```python
from build123d import *

# Parameters (mm, degrees)
CROQUIS1_R                = 3
SALIENTE_EXTRUIR1_DEPTH   = 4
SALIENTE_EXTRUIR1_2_DEPTH = 4
SALIENTE_EXTRUIR1_3_DEPTH = 4
SALIENTE_EXTRUIR1_4_DEPTH = 4
SALIENTE_EXTRUIR2_START   = 3
SALIENTE_EXTRUIR2_DEPTH   = 3
SALIENTE_EXTRUIR3_START   = 3
CROQUIS3_R                = 3
SALIENTE_EXTRUIR3_DEPTH   = 3
CROQUIS5_R                = 1.5
CORTAR_EXTRUIR1_DEPTH     = 13


with BuildPart() as part:
    # Croquis1 → Saliente-Extruir1 (new body)
    with BuildSketch(Plane(origin=(0, 0, 0), x_dir=(1, 0, 0), z_dir=(0, 1, 0))):
        with Locations(Location((-29, 24.5, 0), (0, 0, 270))):
            Circle(CROQUIS1_R)
    extrude(amount=-SALIENTE_EXTRUIR1_DEPTH)



with BuildPart() as body_2:
    # Croquis1 → Saliente-Extruir1 2 (new body)
    with BuildSketch(Plane(origin=(0, 0, 0), x_dir=(1, 0, 0), z_dir=(0, 1, 0))):
        with Locations(Location((-29, -24.5, 0), (0, 0, 270))):
            Circle(CROQUIS1_R)
    extrude(amount=-SALIENTE_EXTRUIR1_2_DEPTH)


with BuildPart() as body_3:
    # Croquis1 → Saliente-Extruir1 3 (new body)
    with BuildSketch(Plane(origin=(0, 0, 0), x_dir=(1, 0, 0), z_dir=(0, 1, 0))):
        with Locations(Location((29, -24.5, 0), (0, 0, 270))):
            Circle(CROQUIS1_R)
    extrude(amount=-SALIENTE_EXTRUIR1_3_DEPTH)


with BuildPart() as body_4:
    # Croquis1 → Saliente-Extruir1 4 (new body)
    with BuildSketch(Plane(origin=(0, 0, 0), x_dir=(1, 0, 0), z_dir=(0, 1, 0))):
        with Locations(Location((29, 24.5, 0), (0, 0, 270))):
            Circle(CROQUIS1_R)
    extrude(amount=-SALIENTE_EXTRUIR1_4_DEPTH)


with BuildPart() as part_1:
    add(part.part)

    add(body_2.part)  # Saliente-Extruir2 merges body 2

    add(body_3.part)  # Saliente-Extruir2 merges body 3

    add(body_4.part)  # Saliente-Extruir2 merges body 4
    # Croquis2 → Saliente-Extruir2 (add)
    with BuildSketch(Plane(origin=(0, 0, 0), x_dir=(1, 0, 0), z_dir=(0, 1, 0)).offset(SALIENTE_EXTRUIR2_START)):
        with BuildLine():
            Line((0, 3.927289505), (-27.063945052, 26.791656877))
            ThreePointArc((-27.063945052, 26.791656877), (-31.291656877, 26.436054948), (-30.936054948, 22.208343123))
            Line((-30.936054948, 22.208343123), (-4.648628393, 0))
            Line((-4.648628393, 0), (-30.936054948, -22.208343123))
            ThreePointArc((-30.936054948, -22.208343123), (-31.291656877, -26.436054948), (-27.063945052, -26.791656877))
            Line((-27.063945052, -26.791656877), (0, -3.927289505))
            Line((0, -3.927289505), (27.063945052, -26.791656877))
            ThreePointArc((27.063945052, -26.791656877), (31.291656877, -26.436054948), (30.936054948, -22.208343123))
            Line((30.936054948, -22.208343123), (4.648628393, 0))
            Line((4.648628393, 0), (30.936054948, 22.208343123))
            ThreePointArc((30.936054948, 22.208343123), (31.291656877, 26.436054948), (27.063945052, 26.791656877))
            Line((27.063945052, 26.791656877), (0, 3.927289505))
        make_face()
    extrude(amount=-SALIENTE_EXTRUIR2_DEPTH)

    # Croquis3 → Saliente-Extruir3 (add)
    with BuildSketch(Plane(origin=(0, 3, 0), x_dir=(1, 0, 0), z_dir=(0, 1, 0)).offset(SALIENTE_EXTRUIR3_START)):
        with Locations(Location((-29, 24.5, 0), (0, 0, 270))):
            Circle(CROQUIS3_R)
        with Locations(Location((-29, -24.5, 0), (0, 0, 270))):
            Circle(CROQUIS3_R)
        with Locations(Location((29, -24.5, 0), (0, 0, 270))):
            Circle(CROQUIS3_R)
        with Locations(Location((29, 24.5, 0), (0, 0, 270))):
            Circle(CROQUIS3_R)
    extrude(amount=-SALIENTE_EXTRUIR3_DEPTH)

    # Croquis5 → Cortar-Extruir1 (cut)
    with BuildSketch(Plane(origin=(0, 6, 0), x_dir=(1, 0, 0), z_dir=(0, 1, 0))):
        with Locations(Location((-29, 24.5, 0), (0, 0, 270))):
            Circle(CROQUIS5_R)
        with Locations(Location((29, 24.5, 0), (0, 0, 270))):
            Circle(CROQUIS5_R)
        with Locations(Location((29, -24.5, 0), (0, 0, 270))):
            Circle(CROQUIS5_R)
        with Locations(Location((-29, -24.5, 0), (0, 0, 270))):
            Circle(CROQUIS5_R)
    extrude(amount=-CORTAR_EXTRUIR1_DEPTH, mode=Mode.SUBTRACT)


solid = part_1.part
```
CAD build for the part. Positions are in the model's coordinates, mm. A direction names the side the tool comes from. Coordinates: 2 decimals unless noted, no trailing zeros. Loops run counter-clockwise (first coordinate to the right, second up) from the corner with the lowest first, then second, coordinate; pieces in that order, holes last. Notation, with made-up numbers: (-25.75, 41.5) - (-11.75, 41.5) arc R25 ccw to (-11.75, 64.5) - close; hole circle Ø8 at (-13.75, 57.25). An arc over 180 degrees is marked (long way). Use CSV: the item, a comma, the result in double quotes. Start each with the question number.
Q1. Probe probe 1 along X at (y, z) = (-1.75, 24.5); probe 2 along Z at (x, y) = (28.5, 3.5); probe 3 along X at (y, z) = (2, -8.5). List the from-to ranges inside material, lowest first. Write a range as from..to.
Q2. Cut at A-A, the plane y = 3.75. List the corners of the cut face in (x, z), then the cut area to 3 significant figures.
Q3. 3-axis set-ups, long thin cutter, end or side, ignore diameter. For faces 5 (the flat face through (-13.343, 1.521, -15.199)), 6 (the flat face through (-13.7, 1.5, 15.5)), 7 (the cylindrical face through (31.03, 1.07, -26.71)): which of +Z, -Z, +X, -X, +Y, -Y reach the whole face in a straight line?
Q4. Drop flat-ended pins along their axis: P1, Ø4, axis at x = 1, y = 3.5, coming from the -Z side; P2, Ø12, axis at x = 3.5, z = -11.5, coming from the +Y side; P3, Ø1, axis at x = -1.5, z = -3, coming from the -Y side. Give the stop position or say it passes through.
Q5. Two-plate mould, pull along X, no slides. Class faces 1 (the cylindrical face through (-31.6, 1.1, 26)), 2 (the flat face through (28, 6, -26)), 3 (the flat face through (-17.976, 1.521, -11.26)), 4 (the flat face through (17.976, 1.521, 11.26)): +X half, -X half, draft (parallel to the pull), parting line (faces both ways), or undercut.
Q6. Cut at B-B, the plane x = 21.5. List the corners of the cut face in (y, z).
Q7. Cut at D-D, the plane z = -15.5. List the corners of the cut face in (x, y).
Here are the results:
1,probe 1,"-32..-30.5, -27.5..-26, 26..27.5, 30.5..32"
1,probe 2,"-27.46..-25.91, -23.09..-21.54, 21.54..23.09, 25.91..27.46"
1,probe 3,"-14.71..-5.41, 5.41..14.71"
2,outline,"circle Ø6 at (-29, -24.5); circle Ø6 at (-29, 24.5); circle Ø6 at (29, -24.5); circle Ø6 at (29, 24.5); hole circle Ø3 at (-29, -24.5); hole circle Ø3 at (-29, 24.5); hole circle Ø3 at (29, -24.5); hole circle Ø3 at (29, 24.5)"
2,area,"84.8 mm2"
3,face 5,"-Z, +Y, -Y"
3,face 6,"+Z, +Y, -Y"
3,face 7,"none"
4,P1,"z = -6.41"
4,P2,"y = 3"
4,P3,"y = 0"
5,face 1,"undercut"
5,face 2,"draft"
5,face 3,"-X half"
5,face 4,"+X half"
6,outline,"(0, -22.09) - (3, -22.09) - (3, -14.24) - (0, -14.24) - close; (0, 14.24) - (3, 14.24) - (3, 22.09) - (0, 22.09) - close"
7,outline,"(-23, 0) - (-13.7, 0) - (-13.7, 3) - (-23, 3) - close; (13.7, 0) - (23, 0) - (23, 3) - (13.7, 3) - close"
